from build123d import *

# Parameters (mm, degrees)
BOSS_EXTRUDE1_DEPTH = 60
CUT_EXTRUDE1_DEPTH  = 7
CUT_EXTRUDE2_REACH  = 72
SKETCH5_W           = 20
SKETCH5_H           = 60
SKETCH6_W           = 23
SKETCH6_H           = 10
SKETCH6_W_2         = 10
SKETCH6_H_2         = 23
BOSS_EXTRUDE3_DEPTH = 60
SKETCH8_R           = 4.1
CUT_EXTRUDE3_DEPTH  = 61
CHAMFER2_SIZE       = 10
BOSS_EXTRUDE4_DEPTH = 7


with BuildPart() as part:
    # Sketch2 → Boss-Extrude1 (new body)
    with BuildSketch(Plane(origin=(0, 0, 0), x_dir=(0, 0, -1), z_dir=(1, 0, 0))):
        with BuildLine():
            Line((0, 40), (-30, 40))
            Line((-30, 40), (-30, -30))
            Line((-30, -30), (40, -30))
            Line((40, -30), (40, 0))
            ThreePointArc((40, 0), (28.284271247, 28.284271247), (0, 40))
        make_face()
        with BuildLine():
            Line((-25, 35), (-25, -25))
            Line((-25, -25), (35, -25))
            Line((35, -25), (35, 0))
            ThreePointArc((35, 0), (24.748737342, 24.748737342), (0, 35))
            Line((0, 35), (-25, 35))
        make_face(mode=Mode.SUBTRACT)
    extrude(amount=BOSS_EXTRUDE1_DEPTH)

    # Sketch4 → Cut-Extrude1 (cut)
    with BuildSketch(Plane(origin=(60, 0, 0), x_dir=(0, 0, -1), z_dir=(1, 0, 0))):
        with BuildLine():
            Line((0, 40), (-7, 40))
            Line((-7, 40), (-7, 35))
            Line((-7, 35), (0, 35))
            ThreePointArc((0, 35), (24.748737342, 24.748737342), (35, 0))
            Line((35, 0), (35, -7))
            Line((35, -7), (40, -7))
            Line((40, -7), (40, 0))
            ThreePointArc((40, 0), (28.284271247, 28.284271247), (0, 40))
        make_face()
    extrude(amount=-CUT_EXTRUDE1_DEPTH, mode=Mode.SUBTRACT)

    # Sketch5 → Cut-Extrude2 (cut, up to next)
    with BuildSketch(Plane.XY.offset(30), mode=Mode.PRIVATE) as cut_extrude2_sk1:
        with Locations((30, 5)):
            Rectangle(SKETCH5_W, SKETCH5_H)
    cut_extrude2_tool1 = extrude(cut_extrude2_sk1.sketch, amount=-CUT_EXTRUDE2_REACH, mode=Mode.PRIVATE) & part.part
    add(cut_extrude2_tool1.solids().sort_by_distance((30, 5, 30))[0], mode=Mode.SUBTRACT)

    # Sketch6 → Boss-Extrude3 (add)
    with BuildSketch(Plane(origin=(60, 0, 0), x_dir=(0, 0, -1), z_dir=(1, 0, 0))):
        with Locations((-18.5, 45)):
            Rectangle(SKETCH6_W, SKETCH6_H)
        with Locations((45, -18.5)):
            Rectangle(SKETCH6_W_2, SKETCH6_H_2)
    extrude(amount=-BOSS_EXTRUDE3_DEPTH)

    # Sketch8 → Cut-Extrude3 (cut, through all)
    with BuildSketch(Plane(origin=(60, 0, 0), x_dir=(0, 0, -1), z_dir=(1, 0, 0))):
        with Locations((-18.5, 42.5)):
            Circle(SKETCH8_R)
        with Locations((42.5, -18.5)):
            Circle(SKETCH8_R)
    extrude(amount=-CUT_EXTRUDE3_DEPTH, mode=Mode.SUBTRACT)

    # Chamfer2
    chamfer2_edges = [part.edges().sort_by_distance(p)[0] for p in [
        (30, -7, -50),
        (30, 50, 7),
    ]]
    chamfer(chamfer2_edges, length=CHAMFER2_SIZE)

    # Sketch9 → Boss-Extrude4 (add)
    with BuildSketch(Plane(origin=(53, 0, 0), x_dir=(0, 0, -1), z_dir=(1, 0, 0))):
        with BuildLine():
            Line((0, 40), (-7, 40))
            Line((-7, 40), (-7, 35))
            Line((-7, 35), (0, 35))
            ThreePointArc((0, 35), (24.748737342, 24.748737342), (35, 0))
            Line((35, 0), (35, -7))
            Line((35, -7), (40, -7))
            Line((40, -7), (40, 0))
            ThreePointArc((40, 0), (28.284271247, 28.284271247), (0, 40))
        make_face()
    extrude(amount=BOSS_EXTRUDE4_DEPTH)


solid = part.part
Could you check a few things on this model? Use its own coordinates, in mm. A direction names the side the tool comes from. Coordinates: 2 decimals unless noted, no trailing zeros. Order: outer loops, then holes, each group sorted by start corner. A loop starts at its lowest first (then second) coordinate and runs counter-clockwise, first axis right, second up. Notation, with made-up numbers: (57.25, 82.25) -> (100.25, 82.25) arc R11 cw to (100.25, 94.25) -> close; hole circle Ø6 at (2.25, 12.5). An arc over 180 degrees is marked (long way). One line per question, with ' | ' between items.
Q1. Thinking about a two-plate mould opening in Z: for faces 1 (the face through (30, 45, 12)), 2 (the face through (0, 4, 26)), 3 (the face through (30.42, 42.68, 22.596)), which applies, pulls with the +Z half, pulls with the -Z half, needs draft (parallel to the pull), parting line crosses it, or undercut?
Return value:
face 1: pulls with the -Z half | face 2: needs draft | face 3: undercut
Q2. On a 3-axis mill with a long thin cutter (end or side, diameter ignored), from which of +Z, -Z, +X, -X, +Y, -Y can I reach the whole of each face in a straight line? I mean faces 4 (the face through (30, 40, 3)), 5 (the face through (30, 50, 24)), 6 (the face through (30, -24, -50)), 7 (the face through (10, 5, 25)), 8 (the face through (20, 5, 28)). Say none if no direction works.
Return value:
face 4: -Z, +X, -X, +Y | face 5: +Z, -Z, +X, -X, +Y | face 6: -Z, +X, -X, +Y, -Y | face 7: +X, -X | face 8: +Z
Q3. I'm going to push flat-ended pins straight in: P1, Ø7.5, axis at x = 42.5, y = -4, coming from the -Z side; P2, Ø6, axis at x = 51.5, y = -1, coming from the -Z side; P3, Ø5, axis at y = -18.5, z = -42.5, coming from the +X side; P4, Ø7.5, axis at x = 42, z = 3, coming from the +Y side. Where does each tip first touch, or does it pass through?
Return value:
P1: z = -40.75 | P2: z = -40 | P3: through | P4: y = 40
Q4. Imagine slicing it at D-D on y = 42.5. Please give me the cut outline in (x, z).
Return value:
outline: (0, 9.5) -> (60, 9.5) -> (60, 14.4) -> (0, 14.4) -> close; (0, 22.6) -> (60, 22.6) -> (60, 30) -> (0, 30) -> close
Q5. Imagine slicing it at A-A on z = -42.5. Please give me the cut outline in (x, y), and give its area (3 significant figures).
Return value:
outline: (0, -30) -> (60, -30) -> (60, -22.6) -> (0, -22.6) -> close; (0, -14.4) -> (60, -14.4) -> (60, -9.5) -> (0, -9.5) -> close | area: 738 mm²
Q6. Imagine slicing it at C-C on x = 33.5. Please give me the cut outline in (y, z).
Return value:
outline: (-30, -50) -> (-17, -50) -> (-7, -40) -> (0, -40) arc R40 ccw to (40, 0) -> (40, 7) -> (50, 17) -> (50, 30) -> (35, 30) -> (35, 0) arc R35 cw to (0, -35) -> (-25, -35) -> (-25, 30) -> (-30, 30) -> close; hole circle Ø8.2 at (-18.5, -42.5); hole circle Ø8.2 at (42.5, 18.5)
Q7. If I drill on L1, parallel to Z at x = 41, y = -3.5; L2, parallel to Y at x = 26, z = 4.5; L3, parallel to Y at x = 25.5, z = 23.5, over which ranges is the centre line in solid material (lowest first)?
Return value:
L1: -40 to -35, 25 to 30 | L2: -30 to -25, 35 to 40 | L3: -30 to -25, 35 to 50
Q8. Imagine slicing it at B-B on y = -18.5. Please give me the cut outline in (x, z), and give its area (3 significant figures).
Return value:
outline: (0, -50) -> (60, -50) -> (60, -46.6) -> (0, -46.6) -> close; (0, -38.4) -> (60, -38.4) -> (60, -35) -> (0, -35) -> close; (0, 25) -> (20, 25) -> (20, 30) -> (0, 30) -> close; (40, 25) -> (60, 25) -> (60, 30) -> (40, 30) -> close | area: 608 mm²
